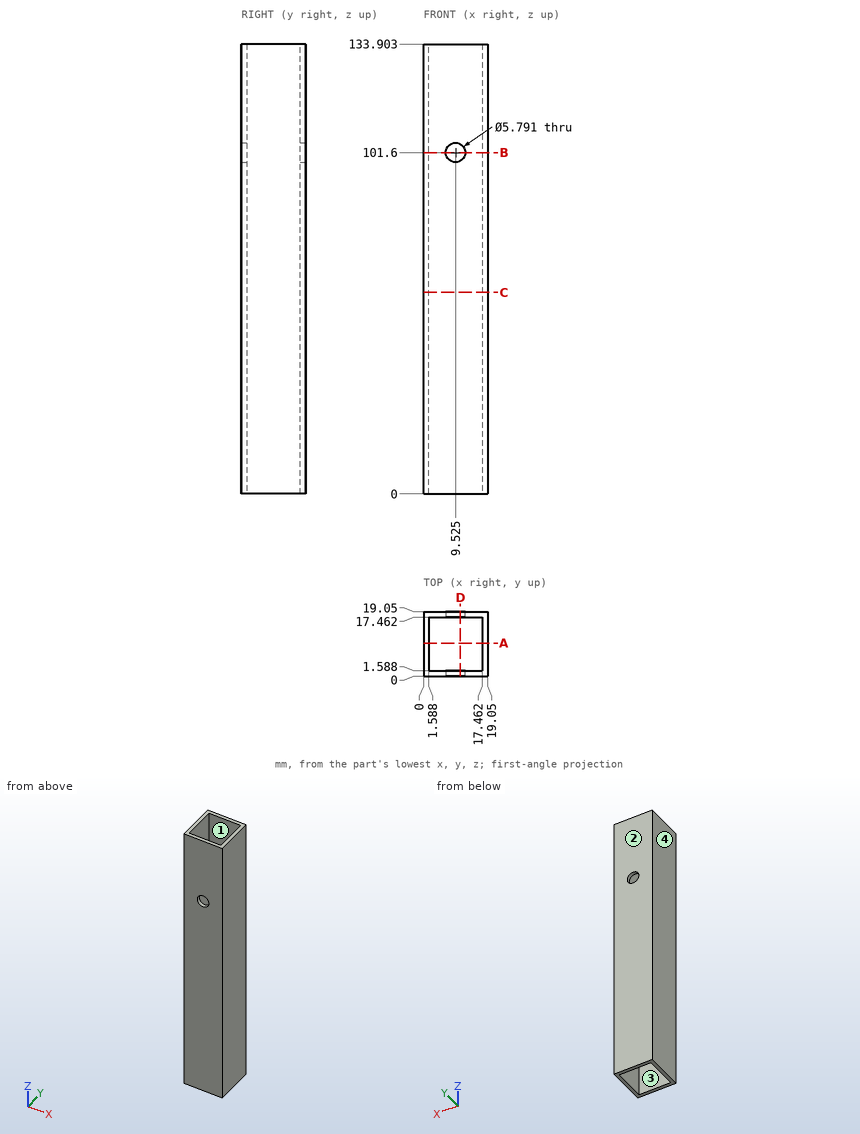
Drawing for the job (mm, zero at the part's lowest x, y, z). Round coordinates to 2 decimals unless told otherwise and drop trailing zeros. Write each loop counter-clockwise with the first axis right and the second up, starting at its lowest first coordinate (ties: lowest second). Pieces come first, ordered by that corner, then holes. Notation, with made-up numbers: M 32.5,87.25 L 73.5,87.25 A9 ccw 73.5,92.25 Z; hole C 70,-20.75 d8. An arc over 180 degrees is marked long. Answer in a Markdown table with one row per item.
1. Saw through at A-A (y = 9.75). List the corners of the cut face in (x, z).
Geometry check:
| item | result |
|---|---|
| outline | M 0,0 L 1.59,0 L 1.59,133.9 L 0,133.9 Z; M 17.46,0 L 19.05,0 L 19.05,133.9 L 17.46,133.9 Z |
2. Flat gauge pins, fed straight in: P1, Ø10, axis at x = 12, y = 9, coming from the -Z side; P2, Ø5, axis at y = 8, z = 78.5, coming from the -X side. Where does each tip first touch, or does it go through?
Geometry check:
| item | result |
|---|---|
| P1 | through |
| P2 | x = 0 |
3. Saw through at C-C (z = 60). List the corners of the cut face in (x, y).
Geometry check:
| item | result |
|---|---|
| outline | M 0,0 L 19.05,0 L 19.05,19.05 L 0,19.05 Z; hole M 1.59,1.59 L 17.46,1.59 L 17.46,17.46 L 1.59,17.46 Z |
4. Saw through at B-B (z = 101.6). List the corners of the cut face in (x, y).
Geometry check:
| item | result |
|---|---|
| outline | M 0,0 L 6.63,0 L 6.63,1.59 L 1.59,1.59 L 1.59,17.46 L 6.63,17.46 L 6.63,19.05 L 0,19.05 Z; M 12.42,0 L 19.05,0 L 19.05,19.05 L 12.42,19.05 L 12.42,17.46 L 17.46,17.46 L 17.46,1.59 L 12.42,1.59 Z |
5. Probe L1, parallel to X at y = 7.25, z = 108. List the from-to ranges inside material, lowest first. Write a range as [from, to].
Geometry check:
| item | result |
|---|---|
| L1 | [0, 1.59], [17.46, 19.05] |
6. Saw through at D-D (x = 11). List the corners of the cut face in (y, z).
Geometry check:
| item | result |
|---|---|
| outline | M 0,0 L 1.59,0 L 1.59,99.11 L 0,99.11 Z; M 0,104.09 L 1.59,104.09 L 1.59,133.9 L 0,133.9 Z; M 17.46,0 L 19.05,0 L 19.05,99.11 L 17.46,99.11 Z; M 17.46,104.09 L 19.05,104.09 L 19.05,133.9 L 17.46,133.9 Z |
7. Mould opens along X. For the marked faces 1, 2, 3 and 4 say: +X half, -X half, draft (parallel to the pull), parting line (faces both ways), or undercut.
Geometry check:
| item | result |
|---|---|
| face 1 | undercut |
| face 2 | draft |
| face 3 | undercut |
| face 4 | -X half |
